Geometry: see drawing. Coordinates: mm, zero at the bounding-box minimum. A direction names the side the tool comes from. Give positions to 0.01 mm unless a question says otherwise; leave off trailing zeros. Loops run counter-clockwise (first coordinate to the right, second up) from the corner with the lowest first, then second, coordinate; pieces in that order, holes last. Notation, with made-up numbers: M 69.25,58 L 103.25,58 A28 cw 103.25,76 Z; hole C 29.25,-29 d3. An arc over 180 degrees is marked long. Answer in a Markdown table with one row per item.
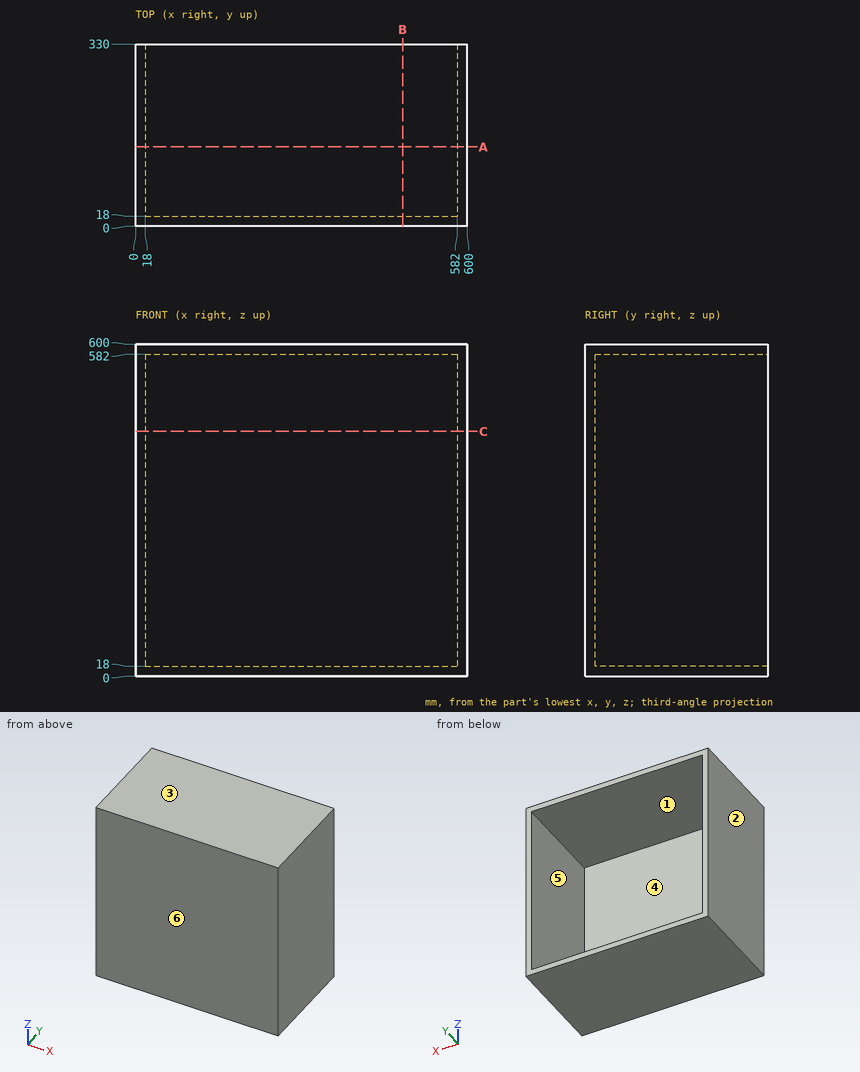
1) Pin query (flat end, axial travel): pin 1 Ø5 at (x, z) = (213.5, 108.5) entering from +Y. Return the tip coordinate at first contact, or that it passes through.
Reply:
| item | result |
|---|---|
| pin 1 | stops at y = 18 |
2) Material intervals for L1, parallel to X at y = 176.5, z = 217.5; L2, parallel to Y at x = 540, z = 129.5, sorted ascending.
Reply:
| item | result |
|---|---|
| L1 | x = 0 to 18, 582 to 600 |
| L2 | y = 0 to 18 |
3) Pull-direction query (Z, two-part tool) for the marked faces 3, 4, 5 and 6; classes: released by +Z, released by -Z, zero draft, split by the parting line, or undercut.
Reply:
| item | result |
|---|---|
| face 3 | released by +Z |
| face 4 | undercut |
| face 5 | undercut |
| face 6 | zero draft |
4) Section C-C, the plane z = 442.5. Return loops of the section in (x, y).
Reply:
| item | result |
|---|---|
| outline | M 0,0 L 600,0 L 600,330 L 582,330 L 582,18 L 18,18 L 18,330 L 0,330 Z |
5) Section A-A, the plane y = 144. Return loops of the section in (x, z).
Reply:
| item | result |
|---|---|
| outline | M 0,0 L 600,0 L 600,600 L 0,600 Z; hole M 18,18 L 582,18 L 582,582 L 18,582 Z |
6) Section B-B, the plane x = 483.5. Return loops of the section in (y, z), then the cut area to 3 significant figures.
Reply:
| item | result |
|---|---|
| outline | M 0,0 L 330,0 L 330,18 L 18,18 L 18,582 L 330,582 L 330,600 L 0,600 Z |
| area | 22,000 mm² |
7) Set-up query: the marked faces 1 and 2. Return all of +Z, -Z, +X, -X, +Y, -Y with unobstructed straight access to the full face (end or side cutting, diameter ignored); none if empty.
Reply:
| item | result |
|---|---|
| face 1 | +Y |
| face 2 | +Z, -Z, -X, +Y, -Y |
